Geometry: final body of the model. Coordinates: model frame, mm. A direction names the side the tool comes from. Give positions to 0.01 mm unless a question says otherwise; leave off trailing zeros. Order: outer loops, then holes, each group sorted by start corner. A loop starts at its lowest first (then second) coordinate and runs counter-clockwise, first axis right, second up. Notation, with made-up numbers: (7.5, 82) -> (54.5, 82) arc R34 cw to (54.5, 114) -> close; hole circle Ø10 at (15.5, 82.25). An arc over 180 degrees is marked (long way). Answer in a Markdown table with one row per item. Add a question column.
Q1. Cut plane A-A on y = 17. Return the cut outline in (x, z), and give its area (3 significant figures).
Q2. Pull-direction query (Z, two-part tool) for faces 5 (the face through (1, 30, 25)), 6 (the face through (2, 39, 26)), 7 (the face through (5, 15.8, 0)), 8 (the face through (0, 29, 26.5)); classes: +Z half, -Z half, draft (parallel to the pull), parting line (faces both ways), or undercut.
Q3. Line query: line 1 along Z through (x, y) = (-5, 37); line 2 along Y through (x, z) = (-3.3, 0); line 3 along X through (y, z) = (14, 0). Output: solid intervals per line, ascending. Write a range as from..to.
Q4. Set-up query: faces 1 (the face through (-14, 37.3, 0)), 2 (the face through (-3.026, 7.05, -0.672)), 3 (the face through (2, 39, -26)), 4 (the face through (-14, 24.3, 0)). Return all of +Z, -Z, +X, -X, +Y, -Y with unobstructed straight access to the full face (end or side cutting, diameter ignored); none if empty.
Q5. Cut plane D-D on x = 0. Return the cut outline in (y, z), and give its area (3 significant figures).
Q6. Cut plane B-B on z = 0. Count the separate pieces of the cut face and the enclosed holes in it, and give its area (3 significant figures).
Q7. Contact query for flat-ended pins moving along their axis: P1, Ø1.6, axis at x = 5.5, z = -25.5, coming from the +Y side; P2, Ø1.7, axis at y = 7, z = 0, coming from the -X side; P3, Ø1.6, axis at x = 22.5, z = 2, coming from the +Y side. Output: stop coordinate, or through.
Q8. Cut plane C-C on z = 8.5. Return the cut outline in (x, y), and give its area (4 significant figures).
from build123d import *

# Parameters (mm, degrees)
SKETCH_1_R               = 4.5
SKETCH_1_R_2             = 3.1
EXTRUDE_1_DEPTH          = 14.3
EXTRUDE_START            = -11.25
EXTRUDE_2_DEPTH          = 11.25
SKETCH_4_W               = 30
SKETCH_4_H               = 50
EXTRUDE_3_DEPTH          = 1.5
SKETCH_5_R               = 1.6
CUT_EXTRUDE_2_DEPTH      = 34.160820255
SKETCH_6_W               = 2.5
SKETCH_6_H               = 50
EXTRUDE_4_DEPTH          = 35
SKETCH_7_W               = 30
SKETCH_7_H               = 13
CUT_EXTRUDE_3_DEPTH      = 10
CUT_EXTRUDE_4_DEPTH      = 59.571665505
CUT_EXTRUDE_4_DEPTH_BACK = 59.571665505
SKETCH_9_R               = 1.55
SKETCH_10_W              = 50
SKETCH_10_H              = 1.5
EXTRUDE_6_DEPTH          = 9
SKETCH_12_W              = 2
SKETCH_12_H              = 50
EXTRUDE_7_DEPTH          = 12
EXTRUDE_8_DEPTH          = 1.5
SKETCH_14_W              = 22
SKETCH_14_H              = 13.5
CUT_EXTRUDE_5_DEPTH      = 78.237555632


with BuildPart() as part:
    # 草图1 → 凸台-拉伸1 (new body)
    with BuildSketch(Plane(origin=(0, 0, 0), x_dir=(1, 0, 0), z_dir=(0, 1, 0))):
        with Locations(Location((0, 0, 0), (0, 0, 270))):
            Circle(SKETCH_1_R)
        with Locations(Location((0, 0, 0), (0, 0, 270))):
            Circle(SKETCH_1_R_2, mode=Mode.SUBTRACT)
    extrude(amount=EXTRUDE_1_DEPTH)

    # 草图2 → 凸台-拉伸2 (add)
    with BuildSketch(Plane(origin=(0, 14.3, 0), x_dir=(1, 0, 0), z_dir=(0, 1, 0)).offset(EXTRUDE_START)):
        with BuildLine():
            Line((2.6, 1.688194302), (2.6, -1.688194302))
            ThreePointArc((2.6, -1.688194302), (3.1, 0), (2.6, 1.688194302))
        make_face()
    extrude(amount=EXTRUDE_2_DEPTH)

    # 草图4 → 凸台-拉伸3 (add)
    with BuildSketch(Plane(origin=(0, 14.3, 0), x_dir=(1, 0, 0), z_dir=(0, 1, 0))):
        Rectangle(SKETCH_4_W, SKETCH_4_H)
    extrude(amount=EXTRUDE_3_DEPTH)

    # 草图5 → 切除-拉伸2 (cut, through all)
    with BuildSketch(Plane(origin=(0, 15.8, 0), x_dir=(1, 0, 0), z_dir=(0, 1, 0))):
        with Locations(Location((0, 0, 0), (0, 0, 270))):
            Circle(SKETCH_5_R)
    extrude(amount=-CUT_EXTRUDE_2_DEPTH, mode=Mode.SUBTRACT)

    # 草图6 → 凸台-拉伸4 (add)
    with BuildSketch(Plane(origin=(0, 15.8, 0), x_dir=(1, 0, 0), z_dir=(0, 1, 0))):
        with Locations((-13.75, 0)):
            Rectangle(SKETCH_6_W, SKETCH_6_H)
    extrude(amount=EXTRUDE_4_DEPTH)

    # 草图7 → 切除-拉伸3 (cut)
    with BuildSketch(Plane(origin=(-12.5, 0, 0), x_dir=(0, 0, -1), z_dir=(1, 0, 0))):
        with Locations((0, 30.8)):
            Rectangle(SKETCH_7_W, SKETCH_7_H)
    extrude(amount=-CUT_EXTRUDE_3_DEPTH, mode=Mode.SUBTRACT)

    # 草图9 → 切除-拉伸4 (cut, two sides: drawn at the far end of the back side and taken through both)
    with BuildSketch(Plane(origin=(0, 0, 0), x_dir=(0, 0, -1), z_dir=(1, 0, 0)).offset(-CUT_EXTRUDE_4_DEPTH_BACK)):
        with Locations((0, 5.3)):
            Circle(SKETCH_9_R)
    extrude(amount=CUT_EXTRUDE_4_DEPTH + CUT_EXTRUDE_4_DEPTH_BACK, mode=Mode.SUBTRACT)

    # 草图10 → 凸台-拉伸6 (add)
    with BuildSketch(Plane(origin=(15, 0, 0), x_dir=(0, 0, -1), z_dir=(1, 0, 0))):
        with Locations((0, 15.05)):
            Rectangle(SKETCH_10_W, SKETCH_10_H)
    extrude(amount=EXTRUDE_6_DEPTH)

    # 草图12 → 凸台-拉伸7 (add)
    with BuildSketch(Plane(origin=(0, 15.8, 0), x_dir=(1, 0, 0), z_dir=(0, 1, 0))):
        with Locations((23, 0)):
            Rectangle(SKETCH_12_W, SKETCH_12_H)
    extrude(amount=EXTRUDE_7_DEPTH)

    # 草图13 → 凸台-拉伸8 (add)
    with BuildSketch(Plane.XY.offset(25)):
        Polygon((24, 27.8), (-12.5, 50.8), (-15, 50.8), (-15, 14.3), (24, 14.3), align=None)
    extrude_8 = extrude(amount=EXTRUDE_8_DEPTH)

    # 镜向2: 凸台-拉伸8 across plane
    add(extrude_8.mirror(Plane.XY))

    # 草图14 → 切除-拉伸5 (cut, through all)
    with BuildSketch(Plane(origin=(0, 0, -26.5), x_dir=(-1, 0, 0), z_dir=(0, 0, -1))):
        with Locations((-13, 44.05)):
            Rectangle(SKETCH_14_W, SKETCH_14_H)
    extrude(amount=-CUT_EXTRUDE_5_DEPTH, mode=Mode.SUBTRACT)


solid = part.part
Completed:
| question | item | result |
|---|---|---|
| 1 | outline | (-15, -26.5) -> (24, -26.5) -> (24, 26.5) -> (-15, 26.5) -> close; hole (-12.5, -25) -> (22, -25) -> (22, 25) -> (-12.5, 25) -> close |
| 1 | area | 342 mm² |
| 2 | face 5 | undercut |
| 2 | face 6 | draft |
| 2 | face 7 | undercut |
| 2 | face 8 | +Z half |
| 3 | line 1 | z = -26.5..-25, 25..26.5 |
| 3 | line 2 | y = 0..3.75, 6.85..15.8 |
| 3 | line 3 | x = -4.5..-3.1, 2.6..4.5 |
| 4 | face 1 | +X, -X |
| 4 | face 2 | -Y |
| 4 | face 3 | +Z, -Z, +X, +Y |
| 4 | face 4 | -X |
| 5 | outline | (0, -4.5) -> (14.3, -4.5) -> (14.3, -26.5) -> (42.92, -26.5) -> (42.92, -25) -> (15.8, -25) -> (15.8, -1.6) -> (14.3, -1.6) -> (14.3, -3.1) -> (0, -3.1) -> close; (0, 3.1) -> (14.3, 3.1) -> (14.3, 1.6) -> (15.8, 1.6) -> (15.8, 25) -> (42.92, 25) -> (42.92, 26.5) -> (14.3, 26.5) -> (14.3, 4.5) -> (0, 4.5) -> close |
| 5 | area | 196 mm² |
| 6 | separate pieces | 5 |
| 6 | enclosed holes | 0 |
| 6 | area | 168 mm² |
| 7 | P1 | stops at y = 37.3 |
| 7 | P2 | stops at x = -4.5 |
| 7 | P3 | stops at y = 27.8 |
| 8 | outline | (-15, 14.3) -> (24, 14.3) -> (24, 27.8) -> (22, 27.8) -> (22, 15.8) -> (-12.5, 15.8) -> (-12.5, 24.3) -> (-15, 24.3) -> close; (-15, 37.3) -> (-12.5, 37.3) -> (-12.5, 50.8) -> (-15, 50.8) -> close |
| 8 | area | 137.5 mm² |
